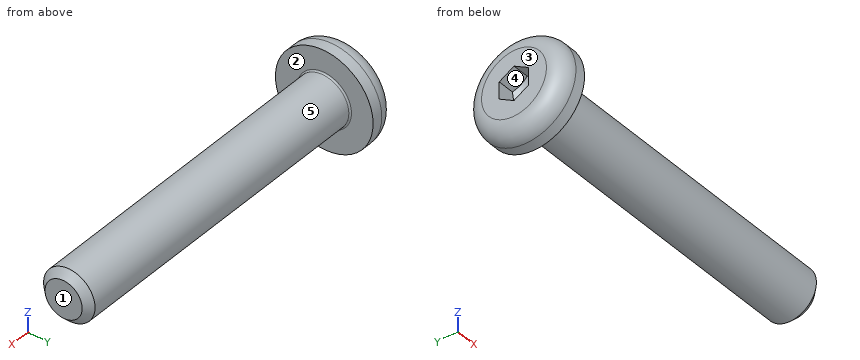
Autodesk Inventor part; units mm, degrees
ref_plane "Work Plane1" through (29, 0, 0) normal (0, -1, 0) x (1, 0, 0)
ref_plane "YZ Plane" through (0, 0, 0) normal (1, 0, 0) x (0, 1, 0)
ref_plane "XZ Plane" through (0, 0, 0) normal (0, 1, 0) x (-1, 0, 0)
sketch "Sketch1" plane through (0, 0, 0) normal (0, 0, 1) x (1, 0, 0)
  line L0 (-0.0677, 0) -> (22.225, 0)
  line L1 (22.225, 0) -> (22.225, 1.7526)
  line L2 (22.225, 1.7526) -> (1.651, 1.7526)
  line L3 (1.651, 1.7526) -> (0.0634, 1.7526)
  line L4 (0.0634, 1.7526) -> (0, 1.7526)
  line L5 (0, 1.7526) -> (0, 3.3274)
  line L6 (0, 3.3274) -> (-1.8542, 3.3274)
  line L7 (-1.8542, 3.3274) -> (-1.8542, 1.1585)
  line L8 (-1.8542, 1.1585) -> (-0.7366, 1.1585)
  line L9 (-0.7366, 1.1585) -> (-0.0677, 0)
  line L10 (-6.67, 0) -> (27.0408, 0)
  line L11 (0, -0.6655) -> (0, 3.9929)
  line L12 (1.651, 1.7526) -> (0, 1.7526) construction
  dimension "d1" = 20.574
  dimension "d2" = 1.5876
  dimension "d3" = 1.8542
  dimension "d4" = 1.1176
  dimension "d5" = 60
  dimension "d6" = 3.5052
  dimension "d7" = 3.5052
  dimension "d8" = 2.317
  dimension "d9" = 6.6548
  dimension "d26" = 22.225
revolve "Body" add sketch "Sketch1" angle 360 about axis through (-0.0677, 0, 0) along (1, 0, 0)
sketch "Sketch2" plane through (-1.8542, 0, 0) normal (-1, 0, 0) x (0, 0, 1)
  circle A0 centre (0, 0) radius 1.1585
  line L0 (0, -4.6584) -> (0, 4.6584)
  line L1 (-4.6584, 0) -> (4.6584, 0)
  line L2 (1.1585, 0) -> (0.5793, -1.0033)
  line L3 (0.5793, -1.0033) -> (-0.5793, -1.0033)
  line L4 (-0.5793, -1.0033) -> (-1.1585, 0)
  line L5 (-1.1585, 0) -> (-0.5793, 1.0033)
  line L6 (-0.5793, 1.0033) -> (0.5793, 1.0033)
  line L7 (0.5793, 1.0033) -> (1.1585, 0)
extrude "Slot" add sketch "Sketch2" against normal up to next contours L7 A0 | A0 L2 | L6 L0 A0 | A0 L0 L3 | L0 L6 A0 | A0 L3 L0 | L4 A0 | A0 L5
fillet "Fillet1" radius 1.1176 1 edges at (-1.8542, -3.3274, 0)
thread "Thread"
chamfer "Chamfer1" distance 0.4869 distance2 0.4869 1 edges at (22.225, -1.7526, 0) measured on face at (22.225, 0.4373, -0.3874)
ref_plane "Work Plane1" through (29, 0, 0) normal (0, -1, 0) x (1, 0, 0)
fillet "Fillet2" radius 0.1 1 edges at (0, -1.7526, 0)
equation "\"d1\" = GEL"
equation "\"d3\" = KOH"
equation "\"d4\" = INTI"
equation "\"d6\" = GD"
equation "\"d7\" = BDM"
equation "\"d8\" = 1.1547 * SW"
equation "\"d9\" = KOD"
equation "\"d26\" = NLG"
equation "\"d30\" = R"
equation "\"d17\" = RR"
equation "\"d13\" = GEL"
equation "\"d15\" = -0.5 * SPD + 0.5 * GD"
equation "\"d16\" = GUL"
equation "\"GD\" = NND"
equation "\"NLG\" = 22.225"
equation "\"GEL\" = 20.574"
equation "\"KOD\" = 6.6548"
equation "\"KOH\" = 1.8542"
equation "\"INTI\" = 1.1176"
equation "\"GAL\" = 1.5875"
equation "\"GUL\" = 0.48692"
equation "\"BDM\" = NND"
equation "\"SW\" = 2.0066"
equation "\"RR\" = 1.1176"
equation "\"SPD\" = GD1"
equation "\"R\" = 0.1"
equation "\"KR\" = 4.0132"
equation "\"GD1\" = 2.53137"
equation "\"THREADDIA\" = 3.5052"
equation "\"FAWI\" = 45deg"
equation "\"KOH1\" = 1.1176"
equation "\"NND\" = 3.5052"
equation "\"TOA\" = 30deg"
equation "\"E0\" = 1.155 * SW"
properties part number "Unbrako - 6 x 7/8" material "Steel, Mild"
Build history of the part. All positions in model axes, mm. Face numbers are marked on the shaded views. A direction names the side the tool comes from. Give positions to 0.01 mm unless a question says otherwise; leave off trailing zeros. Order: outer loops, then holes, each group sorted by start corner. A loop starts at its lowest first (then second) coordinate and runs counter-clockwise, first axis right, second up. Notation, with made-up numbers: M 75,15.5 L 94,15.5 A23 cw 94,39.5 Z; hole C -17.75,-17.5 d11. An arc over 180 degrees is marked long. Use one line per item in the form item = value.
Q1. Pin check, flat tip, straight feed: P1, Ø3, axis at x = 5, y = -1, coming from the +Z side. Stop position of the tip, or through.
Conclusion:
P1 = 1.75
Q2. Wall check: probe 1 along X at (y, z) = (-1.25, 1.5); probe 2 along Y at (x, z) = (8.75, 1.5); probe 3 along X at (y, z) = (-2, -2). Give the ranges that are in metal, low to high.
Conclusion:
probe_1 = -1.85 to 0
probe_2 = -0.91 to 0.91
probe_3 = -1.67 to 0
Q3. Which spindle directions (+Z, -Z, +X, -X, +Y, -Y) get a long thin tool onto all of the face, cutting with end or side? Do the marked faces 1 and 2. Say none if no direction does.
Conclusion:
face_1 = +Z, -Z, +X, +Y, -Y
face_2 = +X
Q4. Slice it at A-A, the plane x = 15.25. Write the cut outline in (y, z), and give its area (3 significant figures).
Conclusion:
outline = C 0,0 d3.51
area = 9.65 mm2
Q5. Pull direction Y, two halves, no side cores. Call the marked faces 3, 4 and 5: released by +Y, released by -Y, zero draft, split by the parting line, or undercut.
Conclusion:
face_3 = zero draft
face_4 = undercut
face_5 = split by the parting line
